The listing builds one solid part. Answer for the finished solid, in the listing's coordinates (mm). A direction names the side the tool comes from. Give positions to 0.01 mm unless a question says otherwise; leave off trailing zeros. Loops run counter-clockwise (first coordinate to the right, second up) from the corner with the lowest first, then second, coordinate; pieces in that order, holes last. Notation, with made-up numbers: M 87,55 L 132,55 A23 cw 132,94 Z; hole C 28.5,35 d9. An arc over 180 degrees is marked long. One line per item, written item: value. Start each with the question number.
Q1. A cutting plane is placed at C-C, the plane z = 25.5. Determine the outline of the cut face in (x, y).
Q2. Consider L1, parallel to X at y = 10, z = 20.25; L2, parallel to X at y = -22, z = 16.5; L3, parallel to Y at x = 15.5, z = 23.75. Determine where each line is inside the solid, lowest interval first.
Q3. Flat-ended cylindrical pins translate along their axes: pin 1 (1 mm diameter, centred on y = 5, z = 18.5, fed in from -X); pin 2 (4 mm diameter, centred on y = 8, z = 15.5, fed in from +X); pin 3 (4 mm diameter, centred on x = -12.5, y = 11.5, fed in from +Z). Find the tip coordinate at first contact, or state that the pin passes through.
Q4. For faces 1 (the flat face through (3, 9.154, 21)), 2 (the flat face through (-12, 12, 20)), 3 (the cylindrical face through (34.247, -0.456, 17.502)), determine the directions among +Z, -Z, +X, -X, +Y, -Y from which every point of the face is accessible in a straight line to the end or side of a thin tool.
Q5. A cutting plane is placed at B-B, the plane y = 3.5. Determine the outline of the cut face in (x, z), and give its area (3 significant figures).
Q6. The mould has two halves that part along Y. Classify faces 4 (the flat face through (3, -30.846, 21)), 5 (the flat face through (3, 14.154, 21)), 6 (the flat face through (-26.985, -11, 21)), 7 (the cylindrical face through (-28.253, -0.236, 17.502)): +Y half, -Y half, draft (parallel to the pull), parting line (faces both ways), or undercut.
Q7. A cutting plane is placed at A-A, the plane x = 0.5. Determine the outline of the cut face in (y, z), and give its area (3 significant figures).
Q8. A cutting plane is placed at D-D, the plane z = 18.75. Determine the outline of the cut face in (x, y).
from build123d import *

# Parameters (mm, degrees)
SKETCH1_W           = 60
SKETCH1_H           = 50
BOSS_EXTRUDE1_DEPTH = 30
SKETCH2_W           = 50
SKETCH2_H           = 40
CUT_EXTRUDE1_DEPTH  = 58.226541049
SKETCH3_W           = 20
SKETCH3_H           = 22.5
CUT_EXTRUDE2_DEPTH  = 5
SKETCH4_W           = 20
SKETCH4_H           = 10
CUT_EXTRUDE3_DEPTH  = 10
SKETCH5_W           = 62.459499436
SKETCH5_H           = 12.5
CUT_EXTRUDE4_DEPTH  = 68.007244418
SKETCH6_R           = 2.5
BOSS_EXTRUDE2_DEPTH = 2.5
BOSS_EXTRUDE3_START = 2.5
SKETCH7_R           = 2.5
BOSS_EXTRUDE3_DEPTH = 2.5


with BuildPart() as part:
    # Sketch1 → Boss-Extrude1 (new body)
    with BuildSketch(Plane.XY):
        with Locations((3.014705882, -10.845588235)):
            Rectangle(SKETCH1_W, SKETCH1_H)
    extrude(amount=BOSS_EXTRUDE1_DEPTH)

    # Sketch2 → Cut-Extrude1 (cut, through all)
    with BuildSketch(Plane.XY.offset(30)):
        with Locations((3.014705882, -10.845588235)):
            Rectangle(SKETCH2_W, SKETCH2_H)
    extrude(amount=-CUT_EXTRUDE1_DEPTH, mode=Mode.SUBTRACT)

    # Sketch3 → Cut-Extrude2 (cut)
    with BuildSketch(Plane(origin=(0, 14.154411765, 0), x_dir=(1, 0, 0), z_dir=(0, 1, 0))):
        with Locations((18.014705882, -11.25)):
            Rectangle(SKETCH3_W, SKETCH3_H)
    extrude(amount=-CUT_EXTRUDE2_DEPTH, mode=Mode.SUBTRACT)

    # Sketch4 → Cut-Extrude3 (cut)
    with BuildSketch(Plane(origin=(0, 14.154411765, 0), x_dir=(1, 0, 0), z_dir=(0, 1, 0))):
        with Locations((-11.985294118, -25)):
            Rectangle(SKETCH4_W, SKETCH4_H)
    extrude(amount=-CUT_EXTRUDE3_DEPTH, mode=Mode.SUBTRACT)

    # Sketch5 → Cut-Extrude4 (cut, through all)
    with BuildSketch(Plane(origin=(0, 14.154411765, 0), x_dir=(1, 0, 0), z_dir=(0, 1, 0))):
        with Locations((2.876613087, -6.25)):
            Rectangle(SKETCH5_W, SKETCH5_H)
    extrude(amount=-CUT_EXTRUDE4_DEPTH, mode=Mode.SUBTRACT)

    # Sketch6 → Boss-Extrude2 (add)
    with BuildSketch(Plane(origin=(33.014705882, 0, 0), x_dir=(0, 0, -1), z_dir=(1, 0, 0))):
        with Locations(Location((-20, -0.345588235, 0), (0, 0, 180))):
            Circle(SKETCH6_R)
    extrude(amount=BOSS_EXTRUDE2_DEPTH)

    # Sketch7 → Boss-Extrude3 (add)
    with BuildSketch(Plane.ZY.offset(26.985294118).offset(BOSS_EXTRUDE3_START)):
        with Locations((20, -0.345588235)):
            Circle(SKETCH7_R)
    extrude(amount=-BOSS_EXTRUDE3_DEPTH)


solid = part.part
Answer block:
1. outline: M -26.99,-35.85 L 33.01,-35.85 L 33.01,14.15 L -1.99,14.15 L -1.99,9.15 L 28.01,9.15 L 28.01,-30.85 L -21.99,-30.85 L -21.99,14.15 L -26.99,14.15 Z
2. L1: -26.99 to -21.99, -1.99 to 8.01, 28.01 to 33.01
2. L2: -26.99 to -21.99, 28.01 to 33.01
2. L3: -35.85 to -30.85, 9.15 to 14.15
3. pin 1: x = -26.99
3. pin 2: x = 33.01
3. pin 3: z = 20
4. face 1: +Z, -Z
4. face 2: +Z, +Y
4. face 3: +X
5. outline: M -26.99,12.5 L -21.99,12.5 L -21.99,30 L -26.99,30 Z; M 28.01,12.5 L 33.01,12.5 L 33.01,30 L 28.01,30 Z
5. area: 175 mm^2
6. face 4: undercut
6. face 5: +Y half
6. face 6: draft
6. face 7: parting line
7. outline: M -35.85,12.5 L -30.85,12.5 L -30.85,30 L -35.85,30 Z; M 9.15,12.5 L 14.15,12.5 L 14.15,30 L 9.15,30 Z
7. area: 175 mm^2
8. outline: M -29.49,-2.51 L -26.99,-2.51 L -26.99,-35.85 L 33.01,-35.85 L 33.01,-2.51 L 35.51,-2.51 L 35.51,1.82 L 33.01,1.82 L 33.01,14.15 L 28.01,14.15 L 28.01,-30.85 L -21.99,-30.85 L -21.99,9.15 L 8.01,9.15 L 8.01,14.15 L -26.99,14.15 L -26.99,1.82 L -29.49,1.82 Z
